Study the drawing (mm; zero at the part's minimum x, y, z) and answer. A direction names the side the tool comes from. Coordinates: 2 decimals unless noted, no trailing zeros. Write each loop counter-clockwise with the first axis right and the second up, starting at its lowest first coordinate (ties: lowest second). Pieces come first, ordered by that corner, then holes. Notation, with made-up numbers: M -19.75,-13.5 L -12.75,-13.5 A23 ccw -12.75,-3.5 Z; hole C -20,85 d3. An arc over 180 degrees is marked long. Answer as CSV lines item,"result". Start each with the question number.
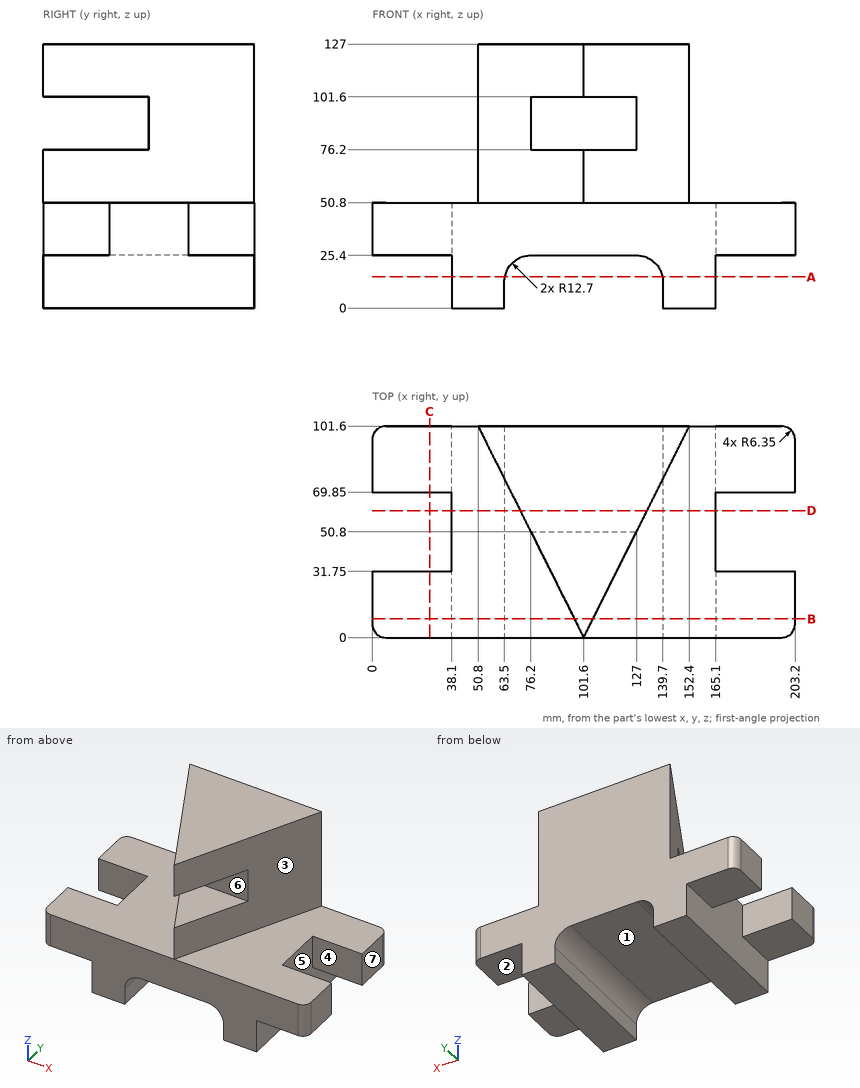
1) Which of the six approach directions +Z, -Z, +X, -X, +Y, -Y give full straight-line access (tool end or side, diameter ignored) to the marked faces 1, 2 and 3?
2) The part is cut by section A-A (z = 15). Determine the outline of the cut face in (x, y).
3) The part is cut by section D-D (y = 61). Determine the outline of the cut face in (x, z).
4) The part is cut by section C-C (x = 27.5). Determine the outline of the cut face in (y, z).
5) Each of these flat-tipped pins is pushed along its axis until it touches: P1, Ø15, axis at x = 108.5, y = 24.5, coming from the -Z side; P2, Ø1.5, axis at x = 55.5, y = 69.5, coming from the +Z side; P3, Ø10, axis at x = 130.5, z = 82.5, coming from the -Y side. Where does it stop, or does it pass through?
6) The part is cut by section B-B (y = 9). Determine the outline of the cut face in (x, z), then the cut area to 3 significant figures.
7) Find the intervals of material crossed by line 1 (Z direction, x = 101.5, y = 25.5); line 2 (Z direction, x = 165, y = 52); line 3 (Z direction, x = 35, y = 93), in increasing order. Write a range as from..to.
8) For a pull along Y with two mould halves and no side action, classify the marked faces 4, 5, 6 and 7 as +Y half, -Y half, draft (parallel to the pull), parting line (faces both ways), or undercut.
Completed:
1,face 1,"-Z, +Y, -Y"
1,face 2,"-Z, +X, +Y, -Y"
1,face 3,"+Z, +X, -Y"
2,outline,"M 38.1,0 L 63.71,0 L 63.71,101.6 L 38.1,101.6 Z; M 139.49,0 L 165.1,0 L 165.1,101.6 L 139.49,101.6 Z"
3,outline,"M 38.1,0 L 63.5,0 L 63.5,12.7 A12.7 cw 76.2,25.4 L 127,25.4 A12.7 cw 139.7,12.7 L 139.7,0 L 165.1,0 L 165.1,50.8 L 132.1,50.8 L 132.1,127 L 71.1,127 L 71.1,50.8 L 38.1,50.8 Z"
4,outline,"M 0,25.4 L 31.75,25.4 L 31.75,50.8 L 0,50.8 Z; M 69.85,25.4 L 101.6,25.4 L 101.6,50.8 L 69.85,50.8 Z"
5,P1,"z = 25.4"
5,P2,"z = 50.8"
5,P3,"y = 50.8"
6,outline,"M 0,25.4 L 38.1,25.4 L 38.1,0 L 63.5,0 L 63.5,12.7 A12.7 cw 76.2,25.4 L 127,25.4 A12.7 cw 139.7,12.7 L 139.7,0 L 165.1,0 L 165.1,25.4 L 203.2,25.4 L 203.2,50.8 L 106.1,50.8 L 106.1,76.2 L 97.1,76.2 L 97.1,50.8 L 0,50.8 Z; M 97.1,101.6 L 106.1,101.6 L 106.1,127 L 97.1,127 Z"
6,area,"6,980 mm²"
7,line 1,"25.4..76.2, 101.6..127"
7,line 2,"0..50.8"
7,line 3,"25.4..50.8"
8,face 4,"undercut"
8,face 5,"undercut"
8,face 6,"-Y half"
8,face 7,"draft"
